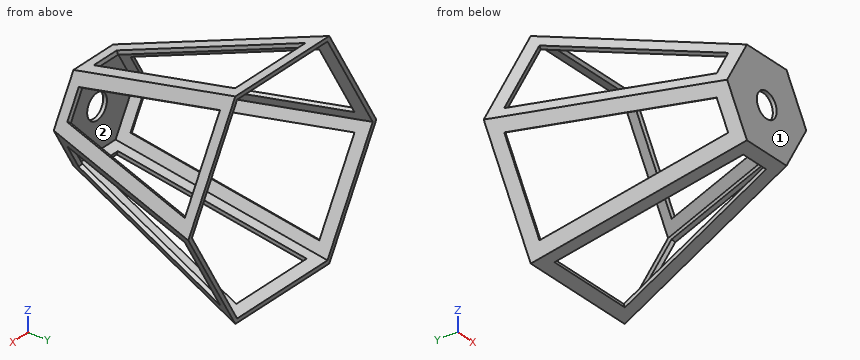
from build123d import *

# Parameters (mm, degrees)
VACIADO1_T            = -3
CORTAR_EXTRUIR1_DEPTH = 3
CORTAR_EXTRUIR2_REACH = 152
CROQUIS4_R            = 10
MATRIZC1_COUNT        = 6


with BuildPart() as part:
    # Croquis2 → Recubrir1 section 0
    with BuildSketch(Plane(origin=(0, 150, 0), x_dir=(-1, 0, 0), z_dir=(0, 1, 0))):
        Polygon((-95, 0), (-47.5, -82.27241336), (47.5, -82.27241336), (95, 0), (47.5, 82.27241336), (-47.5, 82.27241336), align=None)
    # Croquis1 → Recubrir1 section 1
    with BuildSketch(Plane(origin=(0, 0, 0), x_dir=(1, 0, 0), z_dir=(0, 1, 0))):
        Polygon((-40, 0), (-20, -34.641016151), (20, -34.641016151), (40, 0), (20, 34.641016151), (-20, 34.641016151), align=None)
    loft()

    # Vaciado1
    vaciado1_openings = [part.faces().sort_by_distance(p)[0] for p in [
        (0, 150, 0),
    ]]
    offset(amount=VACIADO1_T, openings=vaciado1_openings, kind=Kind.INTERSECTION)

    # Croquis3 → Cortar-Extruir1 (cut)
    with BuildSketch(Plane(origin=(0, -9.992429977, 31.467993476), x_dir=(1, 0, 0), z_dir=(0, -0.302650417, 0.953101634))):
        Polygon((-11.595838701, 20.484117977), (11.595838701, 20.484117977), (35.601132708, 157.865025332), (-35.601132708, 157.865025332), align=None)
    cortar_extruir1 = extrude(amount=-CORTAR_EXTRUIR1_DEPTH, mode=Mode.SUBTRACT)

    # Croquis4 → Cortar-Extruir2 (cut, up to next)
    with BuildSketch(Plane.XZ, mode=Mode.PRIVATE) as cortar_extruir2_sk1:
        Circle(CROQUIS4_R)
    cortar_extruir2_tool1 = extrude(cortar_extruir2_sk1.sketch, amount=-CORTAR_EXTRUIR2_REACH, mode=Mode.PRIVATE) & part.part
    add(cortar_extruir2_tool1.solids().sort_by_distance((0, 0, 0))[0], mode=Mode.SUBTRACT)

    # MatrizC1: Cortar-Extruir1 ×6 about axis
    matrizc1_axis = Axis((0, 0, 0), (0, 1, 0))
    for i in range(1, MATRIZC1_COUNT):
        add(cortar_extruir1.rotate(matrizc1_axis, i * 360 / MATRIZC1_COUNT), mode=Mode.SUBTRACT)


solid = part.part
Check sheet for the modelled part. Datum: model origin and axes. Units: mm. Face numbers are marked on the shaded views. Round coordinates to 2 decimals unless told otherwise and drop trailing zeros. Return JSON: item names as keys, results as strings.
Q1. Draft check along Z on the marked faces 1 and 2. Enter one of: released by +Z, released by -Z, zero draft, split by the parting line, or undercut.
Returned:
{"face 1": "zero draft", "face 2": "undercut"}
Q2. Scan lines: L1, parallel to Z at x = 0, y = 1.5; L2, parallel to X at y = 137.5, z = 72; L3, parallel to Z at x = 41.5, y = 96. Record each from-to range of solid material in increasing order. Write a range as from..to.
Returned:
{"L1": "z = -35.12..-10, 10..35.12", "L2": "x = -48.85..-45.21, 45.21..48.85", "L3": "z = -58.37..-55.57, 55.57..58.37"}
Q3. Cross-section at A-A (x = 0). Give the number of separate pieces and of enclosed holes in the cut face, then the cut area to 3 significant figures.
Returned:
{"separate pieces": "4", "enclosed holes": "0", "area": "252 mm²"}
Q4. Depth check by flat-ended pin: P1, Ø3, axis at x = 18.5, z = -24, coming from the -Y side; P2, Ø1.5, axis at x = -25.5, z = 25, coming from the +Y side. Enter the tip coordinate at first touch or a pass-through.
Returned:
{"P1": "stops at y = 0", "P2": "stops at y = 10.44"}
